Here's how the part is built. I have some questions about the finished solid (model axes, mm). A direction names the side the tool comes from. Round coordinates to 2 decimals unless told otherwise and drop trailing zeros. Write each loop counter-clockwise with the first axis right and the second up, starting at its lowest first coordinate (ties: lowest second). Pieces come first, ordered by that corner, then holes. Notation, with made-up numbers: M 42.5,25.5 L 52.5,25.5 A19 cw 52.5,31.5 Z; hole C 3.5,-9 d1. An arc over 180 degrees is marked long. Write item = value, one per line. Start each with the question number.
(1) I need wall thicknesses on line 1 along Z through (x, y) = (-168.85, 25); line 2 along X through (y, z) = (15.5, -92.5); line 3 along Y through (x, z) = (-168.6, -215). Which ranges of each line are inside material? Lowest first, please.
(2) Will these pins go through, and if not, where does the flat tip stop? pin 1 Ø10 at (x, y) = (-139, 9) entering from +Z; pin 2 Ø4 at (x, y) = (-110.5, 14.5) entering from +Z; pin 3 Ø1.8 at (x, y) = (-164.5, 33.5) entering from -Z.
(3) If we mould it in two halves opening along X, with no side actions, what happens to faces 1 (the flat face through (-170, 25, -108)), 2 (the flat face through (-162, 24, -172)), 3 (the cylindrical face through (-83.81, 24.45, -244.994))? For each: released by +X, released by -X, zero draft, split by the parting line, or undercut.
(4) On a 3-axis mill with a long thin cutter (end or side, diameter ignored), from which of +Z, -Z, +X, -X, +Y, -Y can I reach the whole of each face in a straight line? I mean faces 4 (the cylindrical face through (-83.838, 25.506, 22.994)), 5 (the cylindrical face through (-163.327, 45.986, -50.182)), 6 (the cylindrical face through (-169.01, 24.49, -188.01)). Say none if no direction works.
(5) I want a section at C-C (x = -80.5). List the corners of the cut face in (y, z) for me, and give its area (3 significant figures).
(6) I want a section at A-A (z = -20.5). Give the number of separate pieces and of enclosed holes in the cut face, and give its area (3 significant figures).
Autodesk Inventor part; units mm, degrees
ref_plane "YZ Plane" through (0, 0, 0) normal (1, 0, 0) x (0, 1, 0)
ref_plane "XZ Plane" through (0, 0, 0) normal (0, 1, 0) x (-1, 0, 0)
ref_plane "XY Plane" through (0, 0, 0) normal (0, 0, 1) x (1, 0, 0)
sketch "Sketch1" plane through (0, 0, 0) normal (0, 1, 0) x (-1, 0, 0)
  line L0 (0, 0) -> (170, 0)
  line L1 (170, 0) -> (170, -220)
  line L2 (170, -220) -> (0, -220)
  line L3 (0, -220) -> (0, 0)
  dimension "d0" = 170
  dimension "d1" = 220
extrude "base" add sketch "Sketch1" along normal blind 2
sketch "Sketch2" plane through (0, 2, 0) normal (0, 1, 0) x (1, 0, 0)
  line L0 (0, 0) -> (0, 220)
  line L1 (0, 220) -> (-170, 220)
  line L2 (0, 0) -> (-2, 0)
  line L3 (-2, 0) -> (-2, 220)
  line L4 (-2, 220) -> (0, 220)
  line L5 (0, 220) -> (0, 0)
  line L6 (-170, 220) -> (-170, 0)
  line L7 (-170, 0) -> (-168, 0)
  line L8 (-168, 0) -> (-168, 220)
  line L9 (-168, 220) -> (-170, 220)
  line L10 (-170, 220) -> (-170, 0)
  dimension "d4" = 2
  dimension "d5" = 2
extrude "walls" add sketch "Sketch2" along normal blind 48
sketch "rounded_wall" plane through (0, 0, 0) normal (1, 0, 0) x (0, 0, -1)
  line L0 (0, 0) -> (0, 50)
  line L1 (0, 0) -> (0, 50)
  circle A0 centre (0, 25) radius 25
  circle A1 centre (0, 25) radius 23
  line L2 (220, 0) -> (220, 50)
  line L3 (220, 0) -> (220, 50)
  circle A2 centre (220, 25) radius 25
  line L4 (220, 2) -> (220, 50)
  circle A3 centre (220, 25) radius 23
  point P0 (0, 2)
  point P1 (0, 48)
  point P2 (220, 48)
  dimension "d8" = 46
extrude "rounded_wall_extrusion" add sketch "rounded_wall" against normal blind 170 contours A0 L0 A1 | L2 A3 A2 picked at (-24.1559, 25.9241) picked at (243.9322, 21.4397)
extrude "rounded_wall_side1_extrusion" add sketch "rounded_wall" against normal blind 2 contours A1 L0 | L2 A3 picked at (-13.0084, 23.4205) picked at (235.581, 24.2074)
sketch "rounded_wall_side2" plane through (-170, 0, -220) normal (-1, 0, 0) x (0, 0, 1)
  line L0 (220, 2) -> (220, 48)
  line L1 (220, 48) -> (220, 2)
  arc A0 (220, 2) -> (220, 48) centre (220, 25) ccw
  circle A1 centre (220, 25) radius 23
  line L2 (0, 0) -> (220, 0)
  line L3 (0, 48) -> (0, 2)
  line L4 (0, 48) -> (0, 2)
  arc A2 (0, 48) -> (0, 2) centre (0, 25) ccw
  circle A3 centre (0, 25) radius 23
  point P0 (220, 4.5)
extrude "rounded_wall_side2_extrusion" add sketch "rounded_wall_side2" against normal blind 2 contours L0 A0 | L3 A2
sketch "holes" plane through (0, 25, -220) normal (1, 0, 0) x (0, 0, -1)
  arc A0 (-220, 23) -> (-220, -23) centre (-220, 0) ccw
  line L0 (-220, -23) -> (-179, -23)
  line L1 (-179, -23) -> (-179, 23)
  line L2 (-179, 23) -> (-220, 23)
  line L3 (-220, 23) -> (-220, -23)
  line L4 (-220, -23) -> (0, -23)
  line L5 (0, -23) -> (-41, -23)
  line L6 (-41, -23) -> (-41, 23)
  line L7 (-41, 23) -> (0, 23)
  line L8 (0, 23) -> (0, -23)
  line L9 (-5, -15.5) -> (-36, -15.5)
  line L10 (-36, -15.5) -> (-36, 15.5)
  line L11 (-36, 15.5) -> (-5, 15.5)
  line L12 (-5, 15.5) -> (-5, -15.5)
  arc A1 (0, -23) -> (0, 23) centre (0, 0) ccw
  line L13 (-215, -15.5) -> (-184, -15.5)
  line L14 (-184, -15.5) -> (-184, 15.5)
  line L15 (-184, 15.5) -> (-215, 15.5)
  line L16 (-215, 15.5) -> (-215, -15.5)
  arc A2 (-220, 25) -> (-220, -25) centre (-220, 0) ccw
  point P0 (-20.5, -15.5)
  point P1 (-20.5, -23)
  point P2 (-5, 0)
  point P3 (23, 0)
  point P4 (-215, 0)
  point P5 (-245, 0)
  point P6 (-199.5, -15.5)
  point P7 (-199.5, -23)
  point P8 (-199.5, 0)
  point P9 (-20.5, 0)
  point P10 (-199.5, 23)
  dimension "d15" = 41
  dimension "d16" = 41
  dimension "d17" = 31
  dimension "d18" = 31
  dimension "d19" = 31
  dimension "d20" = 31
hole "shaft_holes" at (0, 25, -20.5) at (0, 25, -199.5) direction (-1, 0, 0) diameter 23 end through all
hole "motor_holes" at (0, 40.5, -5) at (0, 40.5, -36) at (0, 9.5, -5) at (0, 9.5, -36) at (0, 40.5, -184) at (0, 40.5, -215) at (0, 9.5, -215) at (0, 9.5, -184) direction (-1, 0, 0) diameter 3.5 end through all
sketch "Sketch7" plane through (0, 2, 0) normal (0, 1, 0) x (1, 0, 0)
  line L0 (-168, 220) -> (-168, 0)
  line L1 (-2, 220) -> (-2, 0)
  line L2 (-168, 45) -> (-2, 45)
  line L3 (-2, 45) -> (-2, 175)
  line L4 (-2, 175) -> (-168, 175)
  line L5 (-168, 175) -> (-168, 45)
  line L6 (-168, 175) -> (-162, 175)
  line L7 (-162, 175) -> (-162, 169)
  line L8 (-162, 169) -> (-168, 169)
  line L9 (-168, 169) -> (-168, 175)
  line L10 (-168, 45) -> (-162, 45)
  line L11 (-162, 45) -> (-162, 51)
  line L12 (-162, 51) -> (-168, 51)
  line L13 (-168, 51) -> (-168, 45)
  line L14 (-2, 175) -> (-8, 175)
  line L15 (-8, 175) -> (-8, 169)
  line L16 (-8, 169) -> (-2, 169)
  line L17 (-2, 169) -> (-2, 175)
  line L18 (-2, 45) -> (-8, 45)
  line L19 (-8, 45) -> (-8, 51)
  line L20 (-8, 51) -> (-2, 51)
  line L21 (-2, 51) -> (-2, 45)
  point P0 (0, 0)
  point P1 (-168, 110)
  point P2 (-2, 110)
  point P3 (-168, 169)
  point P4 (-162, 175)
  point P5 (-2, 51)
  point P6 (-2, 169)
  dimension "d35" = 130
  dimension "d36" = 6
  dimension "d37" = 6
  dimension "d38" = 6
  dimension "d39" = 6
  dimension "d40" = 6
  dimension "d41" = 6
extrude "columns" add sketch "Sketch7" along normal blind 45 contours L4 L7 L8 L0 | L12 L11 L2 L0 | L4 L1 L16 L15 | L19 L20 L1 L2
sketch "Sketch9" plane through (0, 47, 0) normal (0, 1, 0) x (1, 0, 0)
  line L0 (-8, 175) -> (-2, 175)
  line L1 (-8, 169) -> (-2, 169)
  line L2 (-8, 175) -> (-2, 175)
  line L3 (-2, 175) -> (-2, 169)
  line L4 (-2, 169) -> (-8, 169)
  line L5 (-8, 169) -> (-8, 175)
  line L6 (-8, 51) -> (-2, 51)
  line L7 (-2, 45) -> (-8, 45)
  line L8 (-2, 51) -> (-8, 51)
  line L9 (-8, 51) -> (-8, 45)
  line L10 (-8, 45) -> (-2, 45)
  line L11 (-2, 45) -> (-2, 51)
  line L12 (-162, 51) -> (-162, 45)
  line L13 (-168, 0) -> (-168, 220)
  line L14 (-162, 51) -> (-168, 51)
  line L15 (-168, 51) -> (-168, 45)
  line L16 (-168, 45) -> (-162, 45)
  line L17 (-162, 45) -> (-162, 51)
  line L18 (-162, 175) -> (-168, 175)
  line L19 (-168, 175) -> (-168, 169)
  line L20 (-168, 169) -> (-162, 169)
  line L21 (-162, 169) -> (-162, 175)
  point P0 (0, 0)
  point P1 (-165, 172)
  point P2 (-5, 172)
  point P3 (-5, 48)
  point P4 (-165, 48)
hole "magnet_holders" at (-165, 47, -172) at (-5, 47, -172) at (-5, 47, -48) at (-165, 47, -48) direction (0, -1, 0) diameter 5.5 depth 2
chamfer "chamfers" distance 2 angle 45 2 edges at (-2, 50, -110) (-168, 50, -110)
fillet "fillets" radius 5 2 edges at (-168, 2, -110) (-2, 2, -110)
properties part number "bottom"
Returned:
q1.line_1 = -245 to -211, -188 to -32, -9 to 25
q1.line_2 = -170 to -168, -2 to 0
q1.line_3 = 0 to 7.75, 11.25 to 38.75, 42.25 to 48.6
q2.pin_1 = 22.45
q2.pin_2 = 23.51
q2.pin_3 = -243.82
q3.face_1 = released by -X
q3.face_2 = undercut
q3.face_3 = zero draft
q4.face_4 = none
q4.face_5 = +Y
q4.face_6 = +X, -X
q5.outline = M 0,-220 A25 ccw 50,-220 L 48,-220 A23 cw 2,-220 L 2,0 A23 cw 48,0 L 50,0 A25 ccw 0,0 Z
q5.area = 742 mm²
q6.separate_pieces = 3
q6.enclosed_holes = 0
q6.area = 436 mm²
